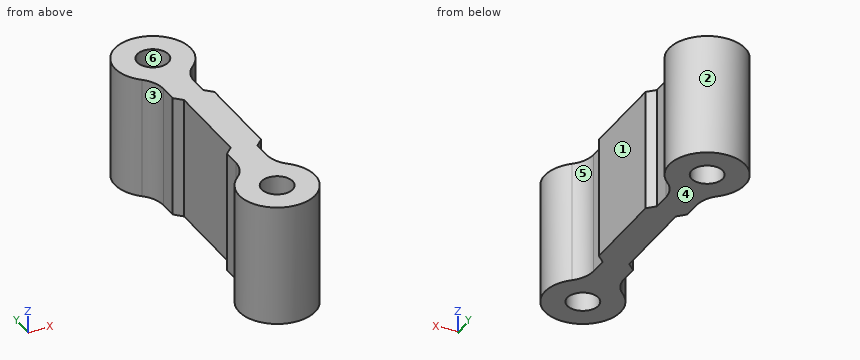
Autodesk Inventor part; units mm, degrees
ref_plane "YZ Plane" through (0, 0, 0) normal (1, 0, 0) x (0, 1, 0)
ref_plane "XZ Plane" through (0, 0, 0) normal (0, 1, 0) x (-1, 0, 0)
ref_plane "XY Plane" through (0, 0, 0) normal (0, 0, 1) x (1, 0, 0)
sketch "Sketch1" plane through (0, 0, 0) normal (0, 0, 1) x (1, 0, 0)
  line L0 (0, 0) -> (0, 12.7) construction
  circle A0 centre (0, 12.7) radius 1.625
  circle A1 centre (0, 12.7) radius 3.9688
  line L1 (-1.5875, -9.0626) -> (1.5875, -9.0626) construction
  line L2 (1.5875, -9.0626) -> (1.5875, 9.0626)
  line L3 (1.5875, 9.0626) -> (-1.5875, 9.0626) construction
  line L4 (-1.5875, 9.0626) -> (-1.5875, -9.0626)
  line L5 (-1.5875, -9.0626) -> (1.5875, 9.0626) construction
  line L6 (1.5875, -9.0626) -> (-1.5875, 9.0626) construction
  circle A2 centre (0, -12.7) radius 1.625
  circle A3 centre (0, -12.7) radius 3.9688
  line L7 (-1.5875, -9.0626) -> (1.5875, -9.0626) construction
  line L8 (-2.3813, -4.7625) -> (-0.7937, -4.7625)
  line L9 (-0.7937, -4.7625) -> (-0.7937, 4.7625)
  line L10 (-0.7937, 4.7625) -> (-2.3813, 4.7625)
  line L11 (-2.3813, 4.7625) -> (-2.3813, -4.7625) construction
  line L12 (-2.3813, -4.7625) -> (-0.7937, 4.7625) construction
  line L13 (-0.7937, -4.7625) -> (-2.3813, 4.7625) construction
  line L14 (0.7937, -4.7625) -> (2.3813, -4.7625)
  line L15 (2.3813, -4.7625) -> (2.3813, 4.7625)
  line L16 (2.3813, 4.7625) -> (0.7937, 4.7625)
  line L17 (0.7937, 4.7625) -> (0.7937, -4.7625) construction
  line L18 (0.7937, -4.7625) -> (2.3813, 4.7625) construction
  line L19 (2.3813, -4.7625) -> (0.7937, 4.7625) construction
  point P0 (-1.5875, 0)
  point P1 (1.5875, 0)
  point P2 (-1.5875, 4.7625)
  point P3 (-1.5875, -4.7625)
  point P4 (1.5875, -4.7625)
  point P5 (1.5875, 4.7625)
  dimension "d2" = 7.9375
  dimension "d0" = 12.7
  dimension "d1" = 3.25
  dimension "d3" = 3.175
  dimension "d6" = 360
  dimension "d8" = 1.5875
  dimension "d9" = 9.525
  dimension "d10" = 1.5875
  dimension "d11" = 9.525
extrude "Extrusion1" add sketch "Sketch1" along normal blind 12.7 contours A1 | A1 L2 A3 L4 L8 L9 L10 | L16 L15 L14 L2 | A3
chamfer "Chamfer1" distance 0.7937 angle 45 4 edges at (-1.5875, 4.7625, 6.35) (1.5875, 4.7625, 6.35) (1.5875, -4.7625, 6.35) (-1.5875, -4.7625, 6.35)
fillet "Fillet1" radius 3.175 4 edges at (1.5875, 9.0626, 6.35) (-1.5875, 9.0626, 6.35) (1.5875, -9.0626, 6.35) (-1.5875, -9.0626, 6.35)
properties part number "Hinge"
Could you check a few things on this model? Use its own coordinates, in mm. Face numbers are marked on the shaded views. A direction names the side the tool comes from. Give positions to 0.01 mm unless a question says otherwise; leave off trailing zeros. Order: outer loops, then holes, each group sorted by start corner. A loop starts at its lowest first (then second) coordinate and runs counter-clockwise, first axis right, second up.
1. Suppose I cut it at A-A (x = 0). List the corners of the cut face in (y, z) for me (3 decimals), plus the area to 3 significant figures.
2. For the marked faces 1, 2 and 3, which set-ups out of +Z, -Z, +X, -X, +Y, -Y let a thin tool reach every point of the face, with its end or its side?
3. I need wall thicknesses on L1, parallel to Y at x = 0, z = 7.75 (3 decimals); L2, parallel to Y at x = 0.5, z = 3.25; L3, parallel to Y at x = -2, z = 4.5. Which ranges of each line are inside material? Lowest first, please.
4. Suppose I cut it at C-C (z = 2). Give the number of separate pieces and of enclosed holes in the cut face, plus the area to 3 significant figures.
5. Suppose I cut it at B-B (y = -12.7). List the corners of the cut face in (x, z) for me (3 decimals), plus the area to 3 significant figures.
6. Suppose I cut it at D-D (x = 3). List the corners of the cut face in (y, z) for me.
7. Will these pins go through, and if not, where does the flat tip stop? P1, Ø4, axis at y = -10, z = 4, coming from the +X side; P2, Ø3, axis at y = -5.5, z = 5, coming from the +X side; P3, Ø1.5, axis at y = 6, z = 8, coming from the +X side.
8. We'd pull the mould along X, two halves only. Please class the marked faces 4, 5 and 6: pulls with the +X half, pulls with the -X half, needs draft (parallel to the pull), parting line crosses it, or undercut.
Solved:
1. outline: (-16.669, 0) - (-14.325, 0) - (-14.325, 12.7) - (-16.669, 12.7) - close; (-11.075, 0) - (11.075, 0) - (11.075, 12.7) - (-11.075, 12.7) - close; (14.325, 0) - (16.669, 0) - (16.669, 12.7) - (14.325, 12.7) - close
1. area: 341 mm2
2. face 1: +Z, -Z, +X
2. face 2: +Z, -Z
2. face 3: +Z, -Z, -X
3. L1: y = -16.669 to -14.325, -11.075 to 11.075, 14.325 to 16.669
3. L2: y = -16.64 to -14.25, -11.15 to 11.15, 14.25 to 16.64
3. L3: y = -16.13 to -8.94, 8.94 to 16.13
4. separate pieces: 1
4. enclosed holes: 2
4. area: 140 mm2
5. outline: (-3.969, 0) - (-1.625, 0) - (-1.625, 12.7) - (-3.969, 12.7) - close; (1.625, 0) - (3.969, 0) - (3.969, 12.7) - (1.625, 12.7) - close
5. area: 59.5 mm2
6. outline: (-15.3, 0) - (-10.1, 0) - (-10.1, 12.7) - (-15.3, 12.7) - close; (10.1, 0) - (15.3, 0) - (15.3, 12.7) - (10.1, 12.7) - close
7. P1: stops at x = 3.91
7. P2: stops at x = 2.38
7. P3: stops at x = 1.89
8. face 4: needs draft
8. face 5: pulls with the +X half
8. face 6: undercut
